The model under review builds one solid part; all positions refer to its coordinate system, in mm. A direction names the side the tool comes from. Give positions to 0.01 mm unless a question says otherwise; leave off trailing zeros. Order: outer loops, then holes, each group sorted by start corner. A loop starts at its lowest first (then second) coordinate and runs counter-clockwise, first axis right, second up. Notation, with made-up numbers: (-7.5, 21.25) - (2.5, 21.25) arc R11 cw to (2.5, 37.25) - close; hole circle Ø7 at (29.5, -7.75). An arc over 180 degrees is marked (long way). Put each result on its own line as item: value.
Autodesk Inventor part; units mm, degrees
ref_plane "YZ Plane" through (0, 0, 0) normal (1, 0, 0) x (0, 1, 0)
ref_plane "XZ Plane" through (0, 0, 0) normal (0, 1, 0) x (-1, 0, 0)
ref_plane "XY Plane" through (0, 0, 0) normal (0, 0, 1) x (1, 0, 0)
sketch "スケッチ1" plane through (0, 0, 0) normal (0, 1, 0) x (-1, 0, 0)
  circle A0 centre (0, 0) radius 3 construction
  circle A1 centre (0, 21.2) radius 3 construction
  line L0 (3, 24.2) -> (-3, 24.2) construction
  line L1 (-3, 24.2) -> (-3, -3) construction
  line L2 (-3, -3) -> (3, -3) construction
  line L3 (3, -3) -> (3, 24.2) construction
  circle A2 centre (0, 21.2) radius 3.5
  circle A3 centre (0, 0) radius 3.5 construction
  line L4 (0, 21.2) -> (-4, 25.2)
  line L5 (-4, 25.2) -> (-4, 30.2)
  circle A4 centre (-4, 30.2) radius 3.5
  line L6 (-0.5, 30.2) -> (-0.5, 26.6497)
  line L7 (-0.5, 26.6497) -> (2.4749, 23.6749)
  line L8 (-7.5, 30.2) -> (-7.5, 23.7503)
  line L9 (-7.5, 23.7503) -> (-2.4749, 18.7251)
  arc A5 (-0.5, 28.3066) -> (0.6716, 25.4782) centre (3.5, 28.3066) ccw
  arc A6 (-7.5, 28.3066) -> (-4.2782, 20.5284) centre (3.5, 28.3066) ccw
  circle A7 centre (-4, 9) radius 3.5
  line L10 (2.4749, 2.4749) -> (0.6716, 4.2782) construction
  arc A8 (-0.5, 7.1066) -> (0.6716, 4.2782) centre (3.5, 7.1066) ccw construction
  line L11 (-10.5, 0.2919) -> (-10.5, -4)
  line L12 (6.5, -4) -> (6.5, 0.2919)
  arc A9 (-10.5, -4) -> (6.5, -4) centre (-2, -4) ccw
  arc A10 (23, 181.2) -> (6.5, 0.2919) centre (1006.5, 0.2919) ccw
  arc A11 (-10.5, 0.2919) -> (-27, 181.2) centre (-1010.5, 0.2919) ccw
  line L13 (6.124, -6.5) -> (-3, -6.5)
  line L14 (-3, -6.5) -> (-3, -9.5)
  line L15 (-3, -9.5) -> (6.124, -9.5)
  line L16 (6.124, -9.5) -> (6.124, -6.5)
  arc A12 (4.4807, -9.5) -> (2.9559, -9.5) centre (3.7183, -8.8529) ccw
  arc A13 (1.0407, -9.5) -> (2.8258, -8.402) centre (1.0407, -7.5) ccw
  line L17 (23, 181.2) -> (-27, 181.2)
  circle A14 centre (-4, 0) radius 3.5
  line L18 (-0.5, 9) -> (-0.5, 0)
  line L19 (-7.5, 0) -> (-7.5, 9)
  line L20 (-4, 3.5) -> (-10.5, 3.5)
  line L21 (-10.5, 3.5) -> (-10.5, -3.5)
  line L22 (-10.5, -3.5) -> (-4, -3.5)
  line L23 (-4, -3.5) -> (-4, 3.5) construction
  arc A15 (-10.5, 6) -> (-7.5, 9) centre (-10.5, 9) ccw
  line L24 (-10.5, 6) -> (-10.6533, 6)
  point P0 (0, -3)
  point P1 (-3, -8)
  point P2 (-10.5, 0)
  point P3 (-7.5, 3.5)
  point P4 (-10.5163, 6)
  dimension "d7" = 7
  dimension "d0" = 6
  dimension "d1" = 6
  dimension "d2" = 21.2
  dimension "d3" = 27.2
  dimension "d4" = 3
  dimension "d5" = 6
  dimension "d6" = 7
  dimension "d8" = 5
  dimension "d9" = 135
  dimension "d10" = 4
  dimension "d11" = 4
  dimension "d12" = 21.2
  dimension "d14" = 6.5
  dimension "d15" = 4
  dimension "d17" = 3
  dimension "d18" = 1
  dimension "d19" = 2
  dimension "d20" = 1000
  dimension "d21" = 50
  dimension "d22" = 160
  dimension "d23" = 3
  dimension "d24" = 6.5
  dimension "d25" = 2.5
extrude "押し出し1" add sketch "スケッチ1" along normal blind 6 contours L9 L8 A6 | A7 A15 L24 A11 L17 A10 L12 A9 L13 L14 L15 L11 L22 A14 L18 | L15 A12 | L15 A13 A12
fillet "フィレット1" radius 1 5 edges at (10.5163, 3, 6) (3, 3, -9.5) (3, 3, -6.5) (-6.124, 3, -6.5) (10.5, 3, -3.5)
sketch "スケッチ2" plane through (0, 6, 0) normal (0, 1, 0) x (1, 0, 0)
  arc A0 (9.4833, 3.5) -> (10.4811, 4.5667) centre (9.4833, 4.5) ccw
  arc A1 (10.4811, 4.5667) -> (-4.4807, 9.5) centre (2, 4) ccw
  arc A2 (-4.4807, 9.5) -> (-2.8258, 8.402) centre (-3.7183, 8.8529) ccw
  arc A3 (-1.0407, 9.5) -> (-2.8258, 8.402) centre (-1.0407, 7.5) ccw
  line L0 (-1.0407, 9.5) -> (2, 9.5)
  arc A4 (3, 8.5) -> (2, 9.5) centre (2, 8.5) ccw
  line L1 (3, 8.5) -> (3, 7.5)
  arc A5 (2, 6.5) -> (3, 7.5) centre (2, 7.5) ccw
  line L2 (2, 6.5) -> (-5.3485, 6.5)
  arc A6 (-5.3485, 6.5) -> (-6.3283, 5.7) centre (-5.3485, 5.5) ccw
  arc A7 (-6.3283, 5.7) -> (-6.5, 4) centre (2, 4) ccw
  line L3 (-6.5, 4) -> (-6.5, -0.2919)
  arc A8 (-23, -181.2) -> (-6.5, -0.2919) centre (-1006.5, -0.2919) ccw
  line L4 (-23, -181.2) -> (27, -181.2)
  arc A9 (10.5242, -7.2472) -> (27, -181.2) centre (1010.5, -0.2919) ccw
  arc A10 (10.5242, -7.2472) -> (9.0363, -6.3813) centre (9.5242, -7.2542) ccw
  arc A11 (9.0363, -6.3813) -> (7.5, -9) centre (10.5, -9) ccw
  arc A12 (0.5, -9) -> (7.5, -9) centre (4, -9) ccw
  line L5 (0.5, -9) -> (0.5, 0)
  arc A13 (4, 3.5) -> (0.5, 0) centre (4, 0) ccw
  line L6 (4, 3.5) -> (9.4833, 3.5)
  arc A14 (7.5, -28.3066) -> (4.2782, -20.5284) centre (-3.5, -28.3066) ccw
  line L7 (7.5, -28.3066) -> (7.5, -30.2)
  arc A15 (0.5, -30.2) -> (7.5, -30.2) centre (4, -30.2) ccw
  line L8 (0.5, -30.2) -> (0.5, -28.3066)
  arc A16 (0.5, -28.3066) -> (-0.6716, -25.4782) centre (-3.5, -28.3066) ccw
  line L9 (-0.6716, -25.4782) -> (-2.4749, -23.6749)
  arc A17 (2.4749, -18.7251) -> (-2.4749, -23.6749) centre (0, -21.2) ccw
  line L10 (2.4749, -18.7251) -> (4.2782, -20.5284)
  arc A18 (-17.0146, -176.2) -> (-2.5039, -45.2) centre (-1006.5, -0.2919) ccw
  arc A19 (6.5039, -45.2) -> (21.0146, -176.2) centre (1010.5, -0.2919) ccw
  arc A20 (-23, -181.2) -> (-6.5, -0.2919) centre (-1006.5, -0.2919) ccw
  arc A21 (10.5242, -7.2472) -> (27, -181.2) centre (1010.5, -0.2919) ccw
  arc A22 (-0.406, -45.2) -> (-2.5039, -45.2) centre (-1.4549, -45.2469) ccw
  arc A23 (6.5039, -45.2) -> (4.406, -45.2) centre (5.4549, -45.2469) ccw
  arc A24 (-2.0146, -176.2) -> (-0.406, -45.2) centre (-1332.9861, -94.346) ccw
  arc A25 (4.406, -45.2) -> (6.0146, -176.2) centre (1336.9861, -94.346) ccw
  line L11 (-17.0146, -176.2) -> (-2.0146, -176.2)
  line L12 (6.0146, -176.2) -> (21.0146, -176.2)
  line L13 (0.5, -9) -> (0.5, 0)
  point P0 (0, 0)
  dimension "d38" = 15
  dimension "d39" = 5
  dimension "d40" = 5
  dimension "d41" = 1.05
  dimension "d42" = 1.05
  dimension "d43" = 15
  dimension "d44" = 15
  dimension "d46" = 5
extrude "押し出し3" cut sketch "スケッチ2" against normal blind 5.7 contours A18 A22 A24 L11 | A19 L12 A25 A23
fillet "フィレット2" radius 2 6 edges at (-17.0146, 3.15, 176.2) (-2.0146, 3.15, 176.2) (6.0146, 3.15, 176.2) (21.0146, 3.15, 176.2) (27, 3, 181.2) (-23, 3, 181.2)
equation "\"d7\" = d6"
equation "\"d12\" = d2"
properties part number "wing" material "ポリカーボネート、スモーク"
(1) Take a section at B-B, the plane z = 155.5. Write out the cut boundary in (x, y).
The answers:
outline: (-18.62, 0) - (22.62, 0) - (22.62, 6) - (17.56, 6) - (17.56, 0.3) - (4.9, 0.3) - (4.9, 6) - (-0.9, 6) - (-0.9, 0.3) - (-13.56, 0.3) - (-13.56, 6) - (-18.62, 6) - close
(2) Take a section at A-A, the plane x = -10. Write out the cut boundary in (y, z).
The answers:
outline: (0, 83.88) - (6, 83.88) - (6, 130.72) - (0.3, 130.72) - (0.3, 176.2) - (6, 176.2) - (6, 181.2) - (0, 181.2) - close
(3) The part is to be moulded in two halves that separate along Z. For faces 1 (the cylindrical face through (-10.414, 2.958, 88.677)), 2 (the flat face through (2, 6, 99)), 3 (the flat face through (8, 0.3, 124)), 4 (the flat face through (13, 3, 176.2)), say which applies: pulls with the +Z half, pulls with the -Z half, needs draft (parallel to the pull), parting line crosses it, or undercut.
The answers:
face 1: pulls with the -Z half
face 2: needs draft
face 3: undercut
face 4: undercut
(4) Wall thickness on L1, parallel to X at y = 4.25, z = 48; L2, parallel to X at y = 1, z = 82.5; L3, parallel to Z at x = 1.5, y = 1: over which ranges is each line inside the solid? List them lowest first.
The answers:
L1: -7.64 to -2.63, -0.31 to 4.31, 6.63 to 11.64
L2: -9.88 to -4.87, 0.45 to 3.55, 8.87 to 13.88
L3: -12.49 to -9.5, -6.5 to -2.45, 11.45 to 18.04, 32.65 to 181.2
(5) Clearance check with flat-ended pins moving along their axes: pin 1 Ø1.8 at (y, z) = (3, 4) entering from +X; pin 2 Ø0.9 at (y, z) = (4, 29) entering from -X; pin 3 Ø2 at (y, z) = (2.5, 125) entering from +X. State where each tip first meets the part, or that it passes through.
The answers:
pin 1: x = 0.5
pin 2: x = -6.93
pin 3: x = 18.43
(6) Take a section at C-C, the plane y = 1.25. Count the separate pieces of the cut face and the enclosed holes in it, then the cut area to 3 significant figures.
The answers:
separate pieces: 1
enclosed holes: 3
area: 2,830 mm^2
(7) For faces 5 (the cylindrical face through (1.5, 2.96, -2.45)), 6 (the cylindrical face through (11.38, 3.19, 108.85)), 7 (the flat face through (1, 3, -9.5)), list the 3-axis set-ups (+Z, -Z, +X, -X, +Y, -Y) from which the entire face can be reached by the end or side of a thin tool; tool diameter is ignored.
The answers:
face 5: +X, +Y, -Y
face 6: +Y
face 7: +Y, -Y
